Build history of the part. All positions in model axes, mm. A direction names the side the tool comes from. Round coordinates to 2 decimals unless told otherwise and drop trailing zeros. Loops run counter-clockwise (first coordinate to the right, second up) from the corner with the lowest first, then second, coordinate; pieces in that order, holes last. Notation, with made-up numbers: (-26.5, 35.5) - (-0.5, 35.5) arc R10 cw to (-0.5, 45.5) - close; hole circle Ø4 at (34, 63). An arc over 180 degrees is marked (long way). Use a Markdown table: item, result.
from build123d import *

# Parameters (mm, degrees)
BOSS_EXTRUDE1_DEPTH = 5.5
CUT_EXTRUDE1_START  = -5.5
CUT_EXTRUDE1_DEPTH  = 5.5


with BuildPart() as part:
    # Sketch1 → Boss-Extrude1 (new body)
    with BuildSketch(Plane.XY):
        with BuildLine():
            Line((-0.226235298, -3.993597074), (-0.311073535, -5.491195977))
            ThreePointArc((-0.311073535, -5.491195977), (1.887741114, 5.165891355), (-3.302674289, -4.397993013))
            Line((-3.302674289, -4.397993013), (-2.401944937, -3.198540373))
            ThreePointArc((-2.401944937, -3.198540373), (1.372902628, 3.757011894), (-0.226235298, -3.993597074))
        make_face()
    extrude(amount=BOSS_EXTRUDE1_DEPTH)

    # Sketch2 → Cut-Extrude1 (cut)
    with BuildSketch(Plane.XY.offset(5.5).offset(CUT_EXTRUDE1_START)):
        with BuildLine():
            Line((-0.5, 4.75), (-0.5, 3.968626967))
            ThreePointArc((-0.5, 3.968626967), (0, 4), (0.5, 3.968626967))
            Line((0.5, 3.968626967), (0.5, 4.75))
            Line((0.5, 4.75), (-0.5, 4.75))
        make_face()
        with BuildLine():
            Line((-3.968626967, 0.5), (-4.75, 0.5))
            Line((-4.75, 0.5), (-4.75, -0.5))
            Line((-4.75, -0.5), (-3.968626967, -0.5))
            ThreePointArc((-3.968626967, -0.5), (-4, 0), (-3.968626967, 0.5))
        make_face()
        with BuildLine():
            Line((4.75, 0.5), (3.968626967, 0.5))
            ThreePointArc((3.968626967, 0.5), (4, 0), (3.968626967, -0.5))
            Line((3.968626967, -0.5), (4.75, -0.5))
            Line((4.75, -0.5), (4.75, 0.5))
        make_face()
    extrude(amount=CUT_EXTRUDE1_DEPTH, mode=Mode.SUBTRACT)


solid = part.part
Q1. Cut at A-A, the plane x = 0. List the corners of the cut face in (y, z), plus the area to 3 significant figures.
Results found:
| item | result |
|---|---|
| outline | (-5.5, 0) - (-4, 0) - (-4, 5.5) - (-5.5, 5.5) - close; (4.75, 0) - (5.5, 0) - (5.5, 5.5) - (4.75, 5.5) - close |
| area | 12.4 mm2 |
Q2. Cut at C-C, the plane y = 0. List the corners of the cut face in (x, z), plus the area to 3 significant figures.
Results found:
| item | result |
|---|---|
| outline | (-5.5, 0) - (-4.75, 0) - (-4.75, 5.5) - (-5.5, 5.5) - close; (4.75, 0) - (5.5, 0) - (5.5, 5.5) - (4.75, 5.5) - close |
| area | 8.25 mm2 |
Q3. Cut at D-D, the plane x = -1.5. List the corners of the cut face in (y, z).
Results found:
| item | result |
|---|---|
| outline | (3.71, 0) - (5.29, 0) - (5.29, 5.5) - (3.71, 5.5) - close |
Q4. Probe line 1 (Y direction, x = 0, z = 4.75); line 2 (X direction, y = 1.75, z = 0.45); line 3 (X direction, y = 3.5, z = 1.7). List the from-to ranges inside material, lowest first.
Results found:
| item | result |
|---|---|
| line 1 | y = -5.5 to -4, 4.75 to 5.5 |
| line 2 | x = -5.21 to -3.6, 3.6 to 5.21 |
| line 3 | x = -4.24 to -1.94, 1.94 to 4.24 |
Q5. Cut at B-B, the plane z = 5. List the corners of the cut face in (x, y).
Results found:
| item | result |
|---|---|
| outline | (-4.75, -0.5) - (-4.75, 0.5) - (-3.97, 0.5) arc R4 cw to (-0.5, 3.97) - (-0.5, 4.75) - (0.5, 4.75) - (0.5, 3.97) arc R4 cw to (3.97, 0.5) - (4.75, 0.5) - (4.75, -0.5) - (3.97, -0.5) arc R4 cw to (-0.23, -3.99) - (-0.31, -5.49) arc R5.5 ccw (long way) to (-3.3, -4.4) - (-2.4, -3.2) arc R4 cw to (-3.97, -0.5) - close |
Q6. Drop flat-ended pins along their axis: pin 1 (0.6 mm diameter, centred on y = 4.5, z = 3.5, fed in from +X); pin 2 (0.9 mm diameter, centred on x = 4, z = 1.5, fed in from -Y); pin 3 (2 mm diameter, centred on y = 2.5, z = 2, fed in from -X). Give the stop position or say it passes through.
Results found:
| item | result |
|---|---|
| pin 1 | stops at x = 3.55 |
| pin 2 | stops at y = -4.2 |
| pin 3 | stops at x = -5.29 |
Q7. Pull direction X, two halves, no side cores. Call faces 4 (the face through (-4.75, 0, 3)), 5 (the face through (2.092, 5.087, 2.712)), 6 (the face through (0.8, 4.1, 5.5)): pulls with the +X half, pulls with the -X half, needs draft (parallel to the pull), parting line crosses it, or undercut.
Results found:
| item | result |
|---|---|
| face 4 | undercut |
| face 5 | parting line crosses it |
| face 6 | needs draft |
Q8. Which spindle directions (+Z, -Z, +X, -X, +Y, -Y) get a long thin tool onto all of the face, cutting with end or side? Do faces 1 (the face through (-2.86, -3.81, 2.71)), 2 (the face through (-3.448, -2.028, 2.712)), 3 (the face through (0.8, 4.1, 0)). Say none if no direction does.
Results found:
| item | result |
|---|---|
| face 1 | +Z, -Z, -Y |
| face 2 | +Z, -Z |
| face 3 | -Z, +X, -X, +Y, -Y |
